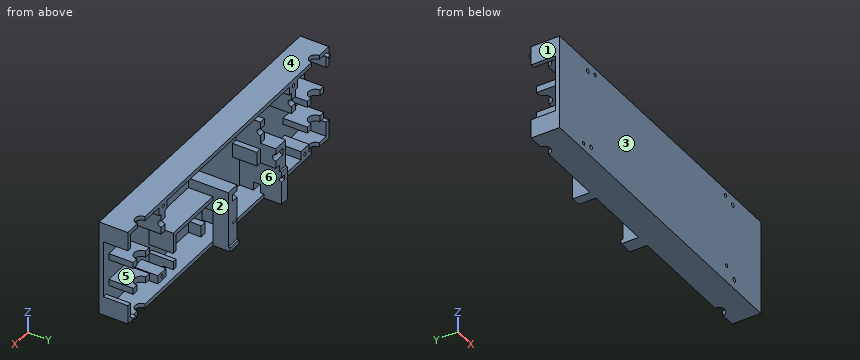
```python
from build123d import *

# Parameters (mm, degrees)
SKETCH_1_W          = 150
SKETCH_1_H          = 45
EXTRUDE_1_DEPTH     = 2
SKETCH_2_W          = 12
SKETCH_2_H          = 3
EXTRUDE_2_DEPTH     = 11.5
SKETCH_4_W          = 3
SKETCH_4_H          = 10
SKETCH_4_W_2        = 2
SKETCH_4_H_2        = 8
EXTRUDE_3_DEPTH     = 11.5
CUT_EXTRUDE_1_REACH = 90.5
SKETCH_5_R          = 2.85
CUT_EXTRUDE_START   = -100.189473
SKETCH_6_R          = 1.6
CUT_EXTRUDE_2_DEPTH = 100.189473
SKETCH_7_W          = 6.45
SKETCH_7_H          = 28.7
EXTRUDE_6_DEPTH     = 7.3
SKETCH_8_W          = 4.5
SKETCH_8_H          = 16
SKETCH_8_W_2        = 6.45
SKETCH_8_H_2        = 2
EXTRUDE_7_DEPTH     = 0.9
CUT_EXTRUDE_START_2 = -3
SKETCH_9_R          = 1.1
SKETCH_9_R_2        = 1.6
CUT_EXTRUDE_3_DEPTH = 37.7
CUT_EXTRUDE_4_REACH = 84.686
SKETCH_10_W         = 4
SKETCH_10_H         = 3.2
CUT_EXTRUDE_8_REACH = 122.235
SKETCH_20_W         = 4
SKETCH_20_H         = 4.9
EXTRUDE_START       = -27
SKETCH_11_W         = 6
SKETCH_11_H         = 4
EXTRUDE_10_DEPTH    = 13.5
CUT_EXTRUDE_5_REACH = 83.254
SKETCH_13_R         = 0.825
CUT_EXTRUDE_START_3 = -32.9
SKETCH_14_R         = 3.25
CUT_EXTRUDE_6_DEPTH = 15.7
EXTRUDE_START_2     = -11.5
SKETCH_17_R         = 0.75
EXTRUDE_12_DEPTH    = 13.5
SKETCH_18_W         = 3
SKETCH_18_H         = 5.5
EXTRUDE_15_DEPTH    = 6
CUT_EXTRUDE_7_REACH = 82.742
SKETCH_19_R         = 1


with BuildPart() as part:
    # 草图1 → 凸台-拉伸1 (new body)
    with BuildSketch(Plane(origin=(0, 0, 0), x_dir=(1, 0, 0), z_dir=(0, 1, 0))):
        Rectangle(SKETCH_1_W, SKETCH_1_H)
    extrude(amount=EXTRUDE_1_DEPTH)

    # 草图2 → 凸台-拉伸2 (add)
    with BuildSketch(Plane(origin=(0, 2, 0), x_dir=(1, 0, 0), z_dir=(0, 1, 0))):
        Polygon((-75, 22.5), (75, 22.5), (75, 13.5), (73, 13.5), (73, 20.5), (1.55, 20.5), (1.55, 8.5), (-0.95, 8.5), (-0.95, 20.5), (-26.6, 20.5), (-26.6, 6.5), (-31.1, 6.5), (-31.1, 20.5), (-73, 20.5), (-73, 13.5), (-75, 13.5), align=None)
        Polygon((75, -22.5), (-75, -22.5), (-75, -13.5), (-73, -13.5), (-73, -20.5), (73, -20.5), (73, -13.5), (75, -13.5), align=None)
        with Locations((-65, -3.8)):
            Rectangle(SKETCH_2_W, SKETCH_2_H)
        with Locations((65, -3.8)):
            Rectangle(SKETCH_2_W, SKETCH_2_H)
        with Locations((-65, 8.9)):
            Rectangle(SKETCH_2_W, SKETCH_2_H)
        with Locations((65, 8.9)):
            Rectangle(SKETCH_2_W, SKETCH_2_H)
    extrude(amount=EXTRUDE_2_DEPTH)

    # 草图4 → 凸台-拉伸3 (add)
    with BuildSketch(Plane(origin=(0, 2, 0), x_dir=(1, 0, 0), z_dir=(0, 1, 0))):
        with Locations((-48.574736579, -11.5)):
            Rectangle(SKETCH_4_W, SKETCH_4_H)
        Polygon((-31.1, 6.5), (-26.6, 6.5), (-26.6, 3.5), (-23.85, 3.5), (-21.25, 3.5), (-21.25, -3.25), (-23.85, -3.25), (-23.85, -16.5), (-26.85, -16.5), (-26.85, -6.2), (-31.1, -6.2), align=None)
        with Locations((48.614736579, -11.5)):
            Rectangle(SKETCH_4_W, SKETCH_4_H)
        Polygon((5.15, 5.5), (11.6, 5.5), (11.6, 0.5), (39.1, 0.5), (39.1, 8.5), (41.1, 8.5), (41.1, -1.5), (11.6, -1.5), (11.6, -6.2), (5.15, -6.2), align=None)
        with Locations((40.1, 16.5)):
            Rectangle(SKETCH_4_W_2, SKETCH_4_H_2)
    extrude(amount=EXTRUDE_3_DEPTH)

    # 切除-拉伸1: up to this face of the body (flat: up to its plane)
    cut_extrude_1_end = Plane(part.part.faces().sort_by_distance((0, 6.75, -22.5))[0])
    # 草图5 → 切除-拉伸1 (cut, up to the picked face)
    with BuildSketch(Plane.XY.offset(22.5), mode=Mode.PRIVATE) as cut_extrude_1_sk1:
        with Locations((-65, 13.5)):
            Circle(SKETCH_5_R)
    cut_extrude_1_tool1 = split(extrude(cut_extrude_1_sk1.sketch, amount=-CUT_EXTRUDE_1_REACH, mode=Mode.PRIVATE), bisect_by=cut_extrude_1_end, keep=Keep.BOTH, mode=Mode.PRIVATE)
    # 草图5 → 切除-拉伸1 (cut, up to the picked face)
    with BuildSketch(Plane.XY.offset(22.5), mode=Mode.PRIVATE) as cut_extrude_1_sk2:
        with Locations((65, 13.5)):
            Circle(SKETCH_5_R)
    cut_extrude_1_tool2 = split(extrude(cut_extrude_1_sk2.sketch, amount=-CUT_EXTRUDE_1_REACH, mode=Mode.PRIVATE), bisect_by=cut_extrude_1_end, keep=Keep.BOTH, mode=Mode.PRIVATE)
    add(cut_extrude_1_tool1.solids().sort_by(Axis((-65, 13.5, 22.5), (0, 0, -1)))[0], mode=Mode.SUBTRACT)
    add(cut_extrude_1_tool2.solids().sort_by(Axis((65, 13.5, 22.5), (0, 0, -1)))[0], mode=Mode.SUBTRACT)

    # 草图6 → 切除-拉伸2 (cut)
    with BuildSketch(Plane(origin=(50.114736579, 0, 0), x_dir=(0, 0, -1), z_dir=(1, 0, 0)).offset(CUT_EXTRUDE_START)):
        with Locations((-11.5, 13.5)):
            Circle(SKETCH_6_R)
    extrude(amount=CUT_EXTRUDE_2_DEPTH, mode=Mode.SUBTRACT)

    # 草图7 → 凸台-拉伸6 (add)
    with BuildSketch(Plane(origin=(0, 13.5, 0), x_dir=(1, 0, 0), z_dir=(0, 1, 0))):
        with Locations((8.375, 8.15)):
            Rectangle(SKETCH_7_W, SKETCH_7_H)
        Polygon((-26.6, 22.5), (-26.6, 3.5), (-23.85, 3.5), (-23.85, -3.25), (-23.85, -6.2), (-31.1, -6.2), (-31.1, 22.5), align=None)
    extrude(amount=EXTRUDE_6_DEPTH)

    # 草图8 → 凸台-拉伸7 (add)
    with BuildSketch(Plane(origin=(0, 20.8, 0), x_dir=(1, 0, 0), z_dir=(0, 1, 0))):
        with Locations((-28.85, 14.5)):
            Rectangle(SKETCH_8_W, SKETCH_8_H)
        with Locations((8.375, 21.5)):
            Rectangle(SKETCH_8_W_2, SKETCH_8_H_2)
    extrude(amount=EXTRUDE_7_DEPTH)

    # 草图9 → 切除-拉伸3 (cut)
    with BuildSketch(Plane(origin=(11.6, 0, 0), x_dir=(0, 0, -1), z_dir=(1, 0, 0)).offset(CUT_EXTRUDE_START_2)):
        with Locations((10.5, 21.7)):
            Circle(SKETCH_9_R)
        with Locations((-1.7, 20.8)):
            Circle(SKETCH_9_R_2)
    extrude(amount=-CUT_EXTRUDE_3_DEPTH, mode=Mode.SUBTRACT)

    # 滑动杆切除-拉伸4: up to this face of the body (flat: up to its plane)
    cut_extrude_4_end = Plane(part.part.faces().sort_by_distance((-31.1, 11.825248606, -7.743924213))[0])
    # 草图10 → 滑动杆切除-拉伸4 (cut, up to the picked face)
    with BuildSketch(Plane(origin=(1.55, 0, 0), x_dir=(0, 0, -1), z_dir=(1, 0, 0)), mode=Mode.PRIVATE) as cut_extrude_4_sk1:
        with Locations((18.5, 10.2)):
            Rectangle(SKETCH_10_W, SKETCH_10_H)
    cut_extrude_4_tool1 = split(extrude(cut_extrude_4_sk1.sketch, amount=-CUT_EXTRUDE_4_REACH, mode=Mode.PRIVATE), bisect_by=cut_extrude_4_end, keep=Keep.BOTH, mode=Mode.PRIVATE)
    add(cut_extrude_4_tool1.solids().sort_by(Axis((1.55, 10.2, -18.5), (-1, 0, 0)))[0], mode=Mode.SUBTRACT)

    # 草图20 → 滑动杆安装切除-拉伸8 (cut, up to next)
    with BuildSketch(Plane(origin=(41.1, 0, 0), x_dir=(0, 0, -1), z_dir=(1, 0, 0)), mode=Mode.PRIVATE) as cut_extrude_8_sk1:
        with Locations((18.5, 11.05)):
            Rectangle(SKETCH_20_W, SKETCH_20_H)
    cut_extrude_8_tool1 = extrude(cut_extrude_8_sk1.sketch, amount=-CUT_EXTRUDE_8_REACH, mode=Mode.PRIVATE) & part.part
    add(cut_extrude_8_tool1.solids().sort_by_distance((41.1, 11.05, -18.5))[0], mode=Mode.SUBTRACT)

    # 草图11 → 螺丝孔凸台-拉伸10 (add)
    with BuildSketch(Plane(origin=(0, 27, 0), x_dir=(1, 0, 0), z_dir=(0, 1, 0)).offset(EXTRUDE_START)):
        with Locations((-48.574736579, -18.5)):
            Rectangle(SKETCH_11_W, SKETCH_11_H)
        with Locations((48.614736579, -18.5)):
            Rectangle(SKETCH_11_W, SKETCH_11_H)
        with Locations((49.55, 14.5)):
            Rectangle(SKETCH_11_W, SKETCH_11_H)
        with Locations((-57.15, 18.5)):
            Rectangle(SKETCH_11_W, SKETCH_11_H)
    extrude(amount=EXTRUDE_10_DEPTH)

    # 草图13 → 螺丝孔切除-拉伸5 (cut, up to next)
    with BuildSketch(Plane.XZ, mode=Mode.PRIVATE) as cut_extrude_5_sk1:
        with Locations(Location((-48.574736579, 19.5, 0), (0, 0, 270))):
            Circle(SKETCH_13_R)
    cut_extrude_5_tool1 = extrude(cut_extrude_5_sk1.sketch, amount=-CUT_EXTRUDE_5_REACH, mode=Mode.PRIVATE) & part.part
    # 草图13 → 螺丝孔切除-拉伸5 (cut, up to next)
    with BuildSketch(Plane.XZ, mode=Mode.PRIVATE) as cut_extrude_5_sk2:
        with Locations(Location((-57.15, -19.5, 0), (0, 0, 270))):
            Circle(SKETCH_13_R)
    cut_extrude_5_tool2 = extrude(cut_extrude_5_sk2.sketch, amount=-CUT_EXTRUDE_5_REACH, mode=Mode.PRIVATE) & part.part
    # 草图13 → 螺丝孔切除-拉伸5 (cut, up to next)
    with BuildSketch(Plane.XZ, mode=Mode.PRIVATE) as cut_extrude_5_sk3:
        with Locations(Location((48.614736579, 19.5, 0), (0, 0, 270))):
            Circle(SKETCH_13_R)
    cut_extrude_5_tool3 = extrude(cut_extrude_5_sk3.sketch, amount=-CUT_EXTRUDE_5_REACH, mode=Mode.PRIVATE) & part.part
    # 草图13 → 螺丝孔切除-拉伸5 (cut, up to next)
    with BuildSketch(Plane.XZ, mode=Mode.PRIVATE) as cut_extrude_5_sk4:
        with Locations(Location((49.55, -14.5, 0), (0, 0, 270))):
            Circle(SKETCH_13_R)
    cut_extrude_5_tool4 = extrude(cut_extrude_5_sk4.sketch, amount=-CUT_EXTRUDE_5_REACH, mode=Mode.PRIVATE) & part.part
    add(cut_extrude_5_tool1.solids().sort_by_distance((-48.574737, 0, 19.5))[0], mode=Mode.SUBTRACT)
    add(cut_extrude_5_tool2.solids().sort_by_distance((-57.15, 0, -19.5))[0], mode=Mode.SUBTRACT)
    add(cut_extrude_5_tool3.solids().sort_by_distance((48.614737, 0, 19.5))[0], mode=Mode.SUBTRACT)
    add(cut_extrude_5_tool4.solids().sort_by_distance((49.55, 0, -14.5))[0], mode=Mode.SUBTRACT)

    # 草图14 → 切除-拉伸6 (cut)
    with BuildSketch(Plane.XY.offset(22.5).offset(CUT_EXTRUDE_START_3)):
        with Locations((-65, 13.5)):
            Circle(SKETCH_14_R)
        with Locations((65, 13.5)):
            Circle(SKETCH_14_R)
    extrude(amount=CUT_EXTRUDE_6_DEPTH, mode=Mode.SUBTRACT)

    # 草图17 → 凸台-拉伸12 (add)
    with BuildSketch(Plane(origin=(0, 13.5, 0), x_dir=(1, 0, 0), z_dir=(0, 1, 0)).offset(EXTRUDE_START_2)):
        with Locations(Location((72.5, 20, 0), (0, 0, 138.189685104))):
            Circle(SKETCH_17_R)
        with Locations(Location((-72.5, -20, 0), (0, 0, 131.810314896))):
            Circle(SKETCH_17_R)
    extrude(amount=EXTRUDE_12_DEPTH)

    # 草图18 → 凸台-拉伸15 (add)
    with BuildSketch(Plane(origin=(0, 2, 0), x_dir=(1, 0, 0), z_dir=(0, 1, 0))):
        with Locations((10.1, 17.75)):
            Rectangle(SKETCH_18_W, SKETCH_18_H)
    extrude(amount=EXTRUDE_15_DEPTH)

    # 草图19 → 切除-拉伸7 (cut, up to next)
    with BuildSketch(Plane(origin=(0, 2, 0), x_dir=(1, 0, 0), z_dir=(0, 1, 0)), mode=Mode.PRIVATE) as cut_extrude_7_sk1:
        with Locations(Location((54.114736579, -18, 0), (0, 0, 270))):
            Circle(SKETCH_19_R)
    cut_extrude_7_tool1 = extrude(cut_extrude_7_sk1.sketch, amount=-CUT_EXTRUDE_7_REACH, mode=Mode.PRIVATE) & part.part
    # 草图19 → 切除-拉伸7 (cut, up to next)
    with BuildSketch(Plane(origin=(0, 2, 0), x_dir=(1, 0, 0), z_dir=(0, 1, 0)), mode=Mode.PRIVATE) as cut_extrude_7_sk2:
        with Locations(Location((-54.074736579, -18, 0), (0, 0, 270))):
            Circle(SKETCH_19_R)
    cut_extrude_7_tool2 = extrude(cut_extrude_7_sk2.sketch, amount=-CUT_EXTRUDE_7_REACH, mode=Mode.PRIVATE) & part.part
    # 草图19 → 切除-拉伸7 (cut, up to next)
    with BuildSketch(Plane(origin=(0, 2, 0), x_dir=(1, 0, 0), z_dir=(0, 1, 0)), mode=Mode.PRIVATE) as cut_extrude_7_sk3:
        with Locations(Location((-51.65, 18, 0), (0, 0, 270))):
            Circle(SKETCH_19_R)
    cut_extrude_7_tool3 = extrude(cut_extrude_7_sk3.sketch, amount=-CUT_EXTRUDE_7_REACH, mode=Mode.PRIVATE) & part.part
    # 草图19 → 切除-拉伸7 (cut, up to next)
    with BuildSketch(Plane(origin=(0, 2, 0), x_dir=(1, 0, 0), z_dir=(0, 1, 0)), mode=Mode.PRIVATE) as cut_extrude_7_sk4:
        with Locations(Location((55.25, 18, 0), (0, 0, 270))):
            Circle(SKETCH_19_R)
    cut_extrude_7_tool4 = extrude(cut_extrude_7_sk4.sketch, amount=-CUT_EXTRUDE_7_REACH, mode=Mode.PRIVATE) & part.part
    add(cut_extrude_7_tool1.solids().sort_by_distance((54.114737, 2, 18))[0], mode=Mode.SUBTRACT)
    add(cut_extrude_7_tool2.solids().sort_by_distance((-54.074737, 2, 18))[0], mode=Mode.SUBTRACT)
    add(cut_extrude_7_tool3.solids().sort_by_distance((-51.65, 2, -18))[0], mode=Mode.SUBTRACT)
    add(cut_extrude_7_tool4.solids().sort_by_distance((55.25, 2, -18))[0], mode=Mode.SUBTRACT)


solid = part.part
```
Source: CAD feature listing. Evaluate the final solid. Frame: model axes, mm. Face numbers are marked on the shaded views. A direction names the side the tool comes from. Give positions to 0.01 mm unless a question says otherwise; leave off trailing zeros. Use a Markdown table: item, result.
Q1. Access query for the marked faces 4, 5 and 6. Directions: +Z, -Z, +X, -X, +Y, -Y. A direction counts if a zero-diameter tool reaches every point of the face in a straight line with its end or side. Return the directions, or none.
A:
| item | result |
|---|---|
| face 4 | +Z, +X, -X, +Y, -Y |
| face 5 | +X, +Y |
| face 6 | +Y |
Q2. Material intervals for line 1 (X direction, y = 0.8, z = -18); line 2 (X direction, y = 5, z = 19.5); line 3 (Z direction, x = 8, y = 4), sorted ascending. Write a range as [from, to].
A:
| item | result |
|---|---|
| line 1 | [-75, -52.65], [-50.65, 54.25], [56.25, 75] |
| line 2 | [-75, -71.94], [-51.57, -49.4], [-47.75, -45.57], [45.61, 47.79], [49.44, 51.61], [73, 75] |
| line 3 | [-22.5, -20.5], [-5.5, 6.2], [20.5, 22.5] |
Q3. Pull-direction query (X, two-part tool) for the marked faces 1, 2 and 3; classes: +X half, -X half, draft (parallel to the pull), parting line (faces both ways), or undercut.
A:
| item | result |
|---|---|
| face 1 | -X half |
| face 2 | undercut |
| face 3 | draft |
Q4. First-contact query: P1, Ø2, axis at x = -22.5, z = -1.5, coming from the +Y side; P2, Ø10, axis at x = 58.5, z = 11.5, coming from the +Y side; P3, Ø0.9, axis at y = 8, z = 4.5, coming from the -X side. Flat tips, straight axial feed; report the tip coordinate or a pass-through.
A:
| item | result |
|---|---|
| P1 | y = 13.5 |
| P2 | y = 2 |
| P3 | x = -71 |
